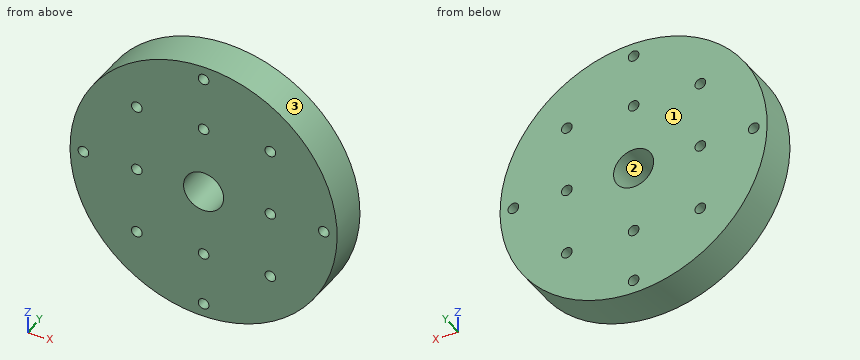
from build123d import *

# Parameters (mm, degrees)
SKETCH1_R           = 50
BOSS_EXTRUDE1_DEPTH = 15
SKETCH2_R           = 7.5
SKETCH2_R_2         = 2
CUT_EXTRUDE1_DEPTH  = 73.284161474


with BuildPart() as part:
    # Sketch1 → Boss-Extrude1 (new body)
    with BuildSketch(Plane(origin=(0, 0, 0), x_dir=(1, 0, 0), z_dir=(0, 1, 0))):
        with Locations(Location((0, 0, 0), (0, 0, 270))):
            Circle(SKETCH1_R)
    extrude(amount=BOSS_EXTRUDE1_DEPTH)

    # Sketch2 → Cut-Extrude1 (cut, through all)
    with BuildSketch(Plane(origin=(0, 15, 0), x_dir=(1, 0, 0), z_dir=(0, 1, 0))):
        with Locations(Location((0, 0, 0), (0, 0, 270))):
            Circle(SKETCH2_R)
        with Locations(Location((45, 0, 0), (0, 0, 270))):
            Circle(SKETCH2_R_2)
        with Locations(Location((0, -45, 0), (0, 0, 270))):
            Circle(SKETCH2_R_2)
        with Locations(Location((0, -25, 0), (0, 0, 270))):
            Circle(SKETCH2_R_2)
        with Locations(Location((25, -25, 0), (0, 0, 270))):
            Circle(SKETCH2_R_2)
        with Locations(Location((-25, -25, 0), (0, 0, 270))):
            Circle(SKETCH2_R_2)
        with Locations(Location((-25, 0, 0), (0, 0, 270))):
            Circle(SKETCH2_R_2)
        with Locations(Location((-45, 0, 0), (0, 0, 270))):
            Circle(SKETCH2_R_2)
        with Locations(Location((-25, 25, 0), (0, 0, 270))):
            Circle(SKETCH2_R_2)
        with Locations(Location((0, 45, 0), (0, 0, 270))):
            Circle(SKETCH2_R_2)
        with Locations(Location((0, 25, 0), (0, 0, 270))):
            Circle(SKETCH2_R_2)
        with Locations(Location((25, 25, 0), (0, 0, 270))):
            Circle(SKETCH2_R_2)
        with Locations(Location((25, 0, 0), (0, 0, 270))):
            Circle(SKETCH2_R_2)
    extrude(amount=-CUT_EXTRUDE1_DEPTH, mode=Mode.SUBTRACT)


solid = part.part
Design review of the part built by this model. Coordinates are the model's own, in mm. Face numbers are marked on the shaded views. Round coordinates to 2 decimals unless told otherwise and drop trailing zeros. Write each loop counter-clockwise with the first axis right and the second up, starting at its lowest first coordinate (ties: lowest second). Pieces come first, ordered by that corner, then holes. Notation, with made-up numbers: (15.25, -19.5) - (64.25, -19.5) arc R13 cw to (64.25, -1.5) - close; hole circle Ø1 at (27.5, 73). An arc over 180 degrees is marked (long way). Use a Markdown table: item, result. Add a question column.
1. We need section C-C (y = 2). Count the separate pieces of the cut face and the enclosed holes in it, then the cut area to 3 significant figures.
2. Clearance check with flat-ended pins moving along their axes: pin 1 (6.5 mm diameter, centred on x = -25, z = 0, fed in from -Y); pin 2 (4 mm diameter, centred on x = -33.5, y = 2, fed in from +Z); pin 3 (6 mm diameter, centred on y = 12, z = 9.5, fed in from -X); pin 4 (5 mm diameter, centred on x = 19, y = 6.5, fed in from -Z). State where each tip first meets the part, or that it passes through.
3. Wall thickness on probe 1 along X at (y, z) = (9, 0); probe 2 along X at (y, z) = (7.5, -1); probe 3 along X at (y, z) = (5, -25): over which ranges is each line inside the solid? List them lowest first.
4. Mouldability with a two-part tool opening along Z and no side actions: class the marked faces 1, 2 and 3 as +Z half, -Z half, draft (parallel to the pull), parting line (faces both ways), or undercut.
5. We need section B-B (x = -45). State the section outline as (y, z) points.
6. We need section A-A (z = 0). State the section outline as (x, y) points.
7. We need section D-D (z = -45). State the section outline as (x, y) points.
Output:
| question | item | result |
|---|---|---|
| 1 | separate pieces | 1 |
| 1 | enclosed holes | 13 |
| 1 | area | 7,530 mm2 |
| 2 | pin 1 | stops at y = 0 |
| 2 | pin 2 | stops at z = 38.83 |
| 2 | pin 3 | stops at x = -49.58 |
| 2 | pin 4 | stops at z = -47.2 |
| 3 | probe 1 | x = -50 to -47, -43 to -27, -23 to -7.5, 7.5 to 23, 27 to 43, 47 to 50 |
| 3 | probe 2 | x = -49.99 to -46.73, -43.27 to -26.73, -23.27 to -7.43, 7.43 to 23.27, 26.73 to 43.27, 46.73 to 49.99 |
| 3 | probe 3 | x = -43.3 to -27, -23 to -2, 2 to 23, 27 to 43.3 |
| 4 | face 1 | draft |
| 4 | face 2 | undercut |
| 4 | face 3 | parting line |
| 5 | outline | (0, -21.79) - (15, -21.79) - (15, -2) - (0, -2) - close; (0, 2) - (15, 2) - (15, 21.79) - (0, 21.79) - close |
| 6 | outline | (-50, 0) - (-47, 0) - (-47, 15) - (-50, 15) - close; (-43, 0) - (-27, 0) - (-27, 15) - (-43, 15) - close; (-23, 0) - (-7.5, 0) - (-7.5, 15) - (-23, 15) - close; (7.5, 0) - (23, 0) - (23, 15) - (7.5, 15) - close; (27, 0) - (43, 0) - (43, 15) - (27, 15) - close; (47, 0) - (50, 0) - (50, 15) - (47, 15) - close |
| 7 | outline | (-21.79, 0) - (-2, 0) - (-2, 15) - (-21.79, 15) - close; (2, 0) - (21.79, 0) - (21.79, 15) - (2, 15) - close |
